Part print with two shaded views. Sizes in mm from the minimum x, y, z corner. A direction names the side the tool comes from. Give positions to 0.01 mm unless a question says otherwise; leave off trailing zeros. Order: outer loops, then holes, each group sorted by start corner. A loop starts at its lowest first (then second) coordinate and runs counter-clockwise, first axis right, second up. Notation, with made-up numbers: M 87,29.25 L 92,29.25 A30 cw 92,64.25 Z; hole C 4.5,-13 d8. An arc over 180 degrees is marked long. Return JSON: item names as keys, results as strings. Group by question number.
1. Slice it at B-B on z = 27.5. List the corners of the cut face in (x, y).
2. Slice it at C-C on y = 14. List the corners of the cut face in (x, z), then the cut area to 3 significant figures.
3. Slice it at A-A on x = 6. List the corners of the cut face in (y, z) (1 decimal), then the cut area to 3 significant figures.
4. 3-axis set-ups, long thin cutter, end or side, ignore diameter. For the marked faces 4, 5, 6 and 7: which of +Z, -Z, +X, -X, +Y, -Y reach the whole face in a straight line?
5. Wall check: probe 1 along Z at (x, y) = (6, 0.4); probe 2 along Z at (x, y) = (6, 0.45) (1 decimal); probe 3 along X at (y, z) = (1.15, 47.5). Give the ranges that are in metal, low to high. Write a range as [from, to].
6. Pin check, flat tips, straight feed: pin 1 (5 mm diameter, centred on x = 4, y = 10, fed in from +Z); pin 2 (6 mm diameter, centred on x = 5.5, z = 47.5, fed in from +Y); pin 3 (2 mm diameter, centred on y = 4, z = 36.5, fed in from -X); pin 4 (5 mm diameter, centred on x = 6, y = 6, fed in from -Z). Stop position of each tip, or through.
7. Two-plate mould, pull along Z, no slides. Class the marked faces 1, 2 and 3: released by +Z, released by -Z, zero draft, split by the parting line, or undercut.
8. Slice it at D-D on z = 51.5. List the corners of the cut face in (x, y).
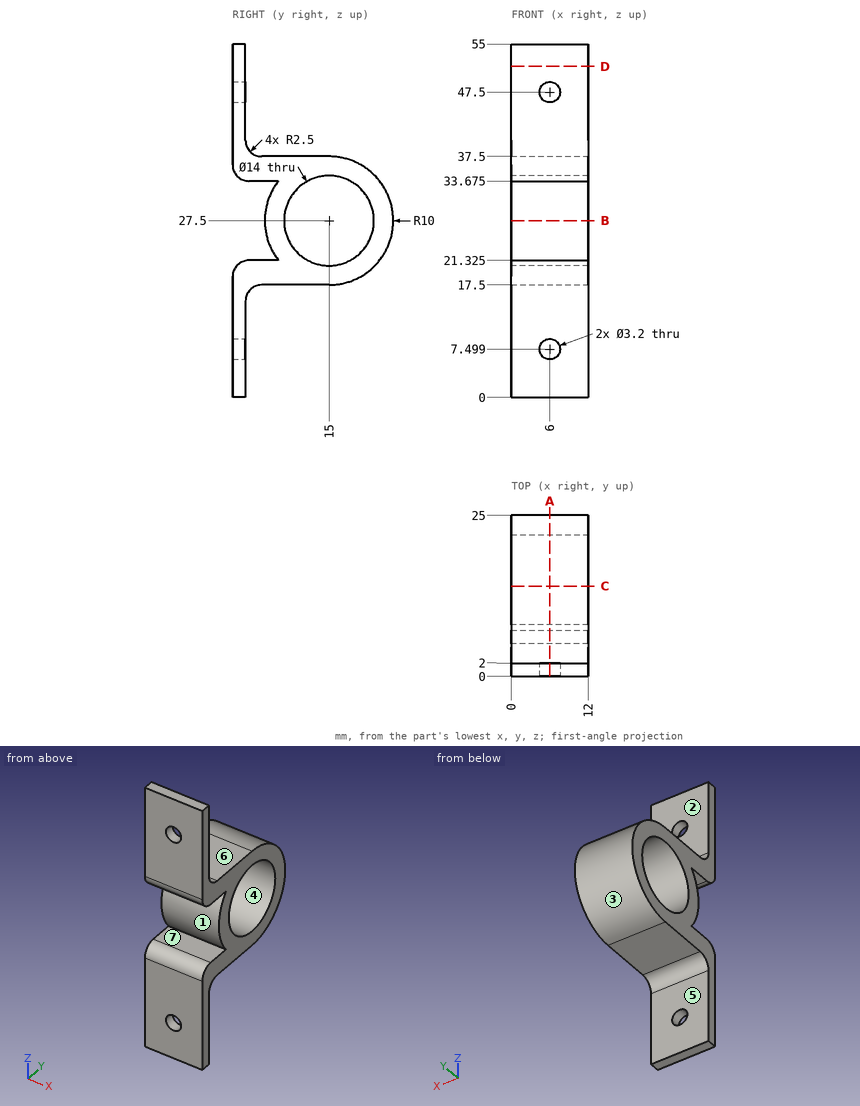
Result:
{
 "1": {"outline": "M 0,5 L 12,5 L 12,8 L 0,8 Z; M 0,22 L 12,22 L 12,25 L 0,25 Z"},
 "2": {"outline": "M 0,17.5 L 12,17.5 L 12,20.57 L 0,20.57 Z; M 0,34.43 L 12,34.43 L 12,37.5 L 0,37.5 Z", "area": "73.7 mm2"},
 "3": {"outline": "M 0,0 L 2,0 L 2,5.9 L 0,5.9 Z; M 0,9.1 L 2,9.1 L 2,15 A2.5 cw 4.5,17.5 L 15,17.5 A10 ccw 15,37.5 L 4.5,37.5 A2.5 cw 2,40 L 2,45.9 L 0,45.9 L 0,36.2 A2.5 ccw 2.5,33.7 L 7.1,33.7 A10 ccw 7.1,21.3 L 2.5,21.3 A2.5 ccw 0,18.8 Z; M 0,49.1 L 2,49.1 L 2,55 L 0,55 Z; hole C 15,27.5 d14", "area": "290 mm2"},
 "4": {"face 4": "+X, -X", "face 5": "-Z, +X, -X, +Y", "face 6": "+Z, +X, -X, +Y", "face 7": "+X, -X, -Y"},
 "5": {"probe 1": "z = [0, 5.9], [9.1, 20.18], [34.82, 45.9], [49.1, 55]", "probe 2": "z = [0, 5.9], [9.1, 20.3], [34.7, 45.9], [49.1, 55]", "probe 3": "x = [0, 4.4], [7.6, 12]"},
 "6": {"pin 1": "stops at z = 37.5", "pin 2": "stops at y = 2", "pin 3": "stops at x = 0", "pin 4": "stops at z = 17.29"},
 "7": {"face 1": "undercut", "face 2": "zero draft", "face 3": "split by the parting line"},
 "8": {"outline": "M 0,0 L 12,0 L 12,2 L 0,2 Z"}
}
